Can you work these out from the model? Positions are in its coordinate system, mm. A direction names the side the tool comes from. Round coordinates to 2 decimals unless told otherwise and drop trailing zeros. Loops run counter-clockwise (first coordinate to the right, second up) from the corner with the lowest first, then second, coordinate; pieces in that order, holes last. Notation, with made-up numbers: M 50.25,44.5 L 59.25,44.5 A20 cw 59.25,56.5 Z; hole C -29.75,-12.5 d2. An arc over 180 degrees is marked long. Return JSON: item names as keys, results as strings.
Autodesk Inventor part; units mm, degrees
ref_plane "YZ Plane" through (0, 0, 0) normal (1, 0, 0) x (0, 1, 0)
ref_plane "XZ Plane" through (0, 0, 0) normal (0, 1, 0) x (-1, 0, 0)
ref_plane "XY Plane" through (0, 0, 0) normal (0, 0, 1) x (1, 0, 0)
sketch "Sketch1" plane through (0, 0, 0) normal (0, 1, 0) x (-1, 0, 0)
  line L0 (-11.5541, -25.4) -> (11.5541, -25.4)
  line L1 (11.5541, -25.4) -> (11.5541, 25.4)
  line L2 (11.5541, 25.4) -> (-11.5541, 25.4)
  line L3 (-11.5541, 25.4) -> (-11.5541, -25.4)
  line L4 (-11.5541, -25.4) -> (11.5541, 25.4) construction
  line L5 (11.5541, -25.4) -> (-11.5541, 25.4) construction
  line L6 (-43.5634, -12.35) -> (-11.5541, -12.35)
  line L7 (-11.5541, -12.35) -> (-11.5541, 12.35)
  line L8 (-11.5541, 12.35) -> (-43.5634, 12.35)
  line L9 (-43.5634, 12.35) -> (-43.5634, -12.35)
  line L10 (-43.5634, -12.35) -> (-11.5541, 12.35) construction
  line L11 (-11.5541, -12.35) -> (-43.5634, 12.35) construction
  point P0 (0, 0)
  point P1 (-27.5588, 0)
  dimension "d0" = 50.8
extrude "Extrusion1" add sketch "Sketch1" along normal mid plane 1.5875
sketch "Sketch2" plane through (43.5634, -0.7937, -12.35) normal (1, 0, 0) x (0, 0, -1)
  line L0 (-4.8431, -19.1223) -> (-18.9376, -19.1223)
  line L1 (-18.9376, -19.1223) -> (-18.9376, 1.5598)
  line L2 (-18.9376, 1.5598) -> (-4.8431, 1.5598)
  line L3 (-4.8431, 1.5598) -> (-4.8431, -19.1223)
  line L4 (-4.8431, -19.1223) -> (-18.9376, 1.5598) construction
  line L5 (-18.9376, -19.1223) -> (-4.8431, 1.5598) construction
  circle A0 centre (-11.8904, -8.7813) radius 1.8384
  point P0 (-12.35, 0.7937)
extrude "Extrusion2" add sketch "Sketch2" along normal blind 1.5875
properties part number "ultrasonic_sensor_ho"
Q1. Suppose I cut it at B-B, the plane x = 38. Please give me the cut outline in (y, z), plus the area to 3 significant figures.
Results:
{"outline": "M -0.79,-12.35 L 0.79,-12.35 L 0.79,12.35 L -0.79,12.35 Z", "area": "39.2 mm2"}
Q2. If I drill on line 1 along X through (y, z) = (-4, -7); line 2 along Y through (x, z) = (36.5, 3), over which ranges is the centre line in solid material (lowest first)?
Results:
{"line 1": "x = 43.56 to 45.15", "line 2": "y = -0.79 to 0.79"}
Q3. I'm going to push flat-ended pins straight in: pin 1 Ø1.3 at (x, z) = (44.5, -3) entering from +Y; pin 2 Ø3 at (y, z) = (-9.57, -0.46) entering from +X; pin 3 Ø1.3 at (y, z) = (0, 18.5) entering from +X; pin 4 Ø1 at (x, z) = (35.5, -3.5) entering from -Y. Where does each tip first touch, or does it pass through?
Results:
{"pin 1": "stops at y = 0.77", "pin 2": "passes through", "pin 3": "stops at x = 11.55", "pin 4": "stops at y = -0.79"}
Q4. Suppose I cut it at C-C, the plane y = -14.25. Please give me the cut outline in (x, z).
Results:
{"outline": "M 43.56,-7.51 L 45.15,-7.51 L 45.15,6.59 L 43.56,6.59 Z"}
Q5. On a 3-axis mill with a long thin cutter (end or side, diameter ignored), from which of +Z, -Z, +X, -X, +Y, -Y can I reach the whole of each face in a straight line? I mean faces 1 (the flat face through (43.563, -12, 0)), 2 (the flat face through (27, 0, 12.35)), 3 (the flat face through (11.554, 0, -19)). Say none if no direction works.
Results:
{"face 1": "+Z, -Z, -X, -Y", "face 2": "+Z, +X, +Y, -Y", "face 3": "-Z, +X, +Y, -Y"}
